Geometry check sheet. Reference: the model listing, model coordinates, mm. Coordinates: 2 decimals unless noted, no trailing zeros. Order: outer loops, then holes, each group sorted by start corner. A loop starts at its lowest first (then second) coordinate and runs counter-clockwise, first axis right, second up.
```python
from build123d import *

# Parameters (mm, degrees)
F2_DEPTH = 12
F3_W     = 392
F3_H     = 368
F3_W_2   = 35
F3_H_2   = 13
F4_DEPTH = 12
F5_R     = 30
F6_R     = 14.99999


# Not quite as in the source:
# - a fillet or chamfer is up to 0.001 mm smaller than in the source, because OpenCascade refuses the exact size
# - a feature names something its author has since deleted; it is built from what else it names


with BuildPart() as f2:
    # F1 (on Front) → F2 (new body)
    with BuildSketch(Plane.XZ):
        Polygon((256, -284), (256, 284), (-256, 284), (-256, -284), (-136, -284), (-136, -254), (136, -254), (136, -284), align=None)
    extrude(amount=F2_DEPTH)

    # F3 (on face) → F4 (cut, through all)
    with BuildSketch(Plane.XZ.offset(12)):
        with Locations((0, 60)):
            Rectangle(F3_W, F3_H)
        with Locations((0, -195.5)):
            Rectangle(F3_W_2, F3_H_2)
    extrude(amount=-F4_DEPTH, mode=Mode.SUBTRACT)

    # F5
    f5_edges = [f2.edges().sort_by_distance(p)[0] for p in [
        (-196, -6, -124),
        (-196, -6, 244),
        (196, -6, 244),
        (196, -6, -124),
    ]]
    fillet(f5_edges, radius=F5_R)

    # F6 (radius 15 in the source; OpenCascade refuses exactly that, so slightly less here)
    f6_edges = [f2.edges().sort_by_distance(p)[0] for p in [
        (-136, -6, -284),
        (-136, -6, -254),
        (136, -6, -284),
        (136, -6, -254),
    ]]
    fillet(f6_edges, radius=F6_R)


solid = f2.part
```
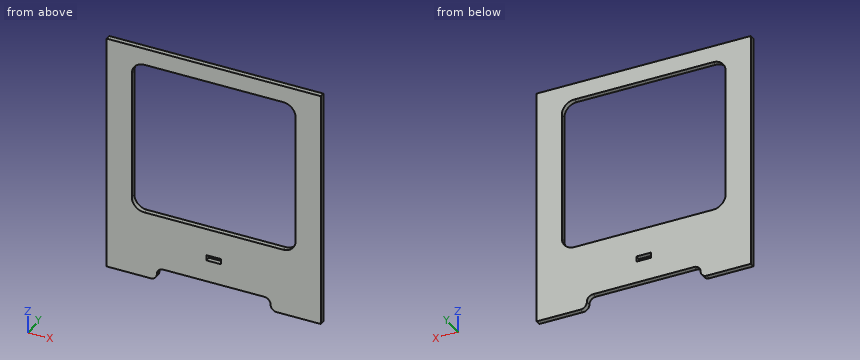
Item 1: Sectioned sample at D-D (x = 1). Record the cut outline in (y, z), and give its area (3 significant figures).
Item 2: Sectioned sample at B-B (y = -7.5). Give the number of separate pieces and of enclosed holes in the cut face, and give its area (3 significant figures).
Item 3: Sectioned sample at A-A (x = 65). Record the cut outline in (y, z), and give its area (3 significant figures).
Item 4: Sectioned sample at C-C (z = 173). Record the cut outline in (x, y).
Item 5: Thickness scan on line 1 along Z through (x, y) = (-18.5, -8); line 2 along X through (y, z) = (-1, 33.5); line 3 along Z through (x, y) = (-10.5, -11). Record the ranges inside material, lowest first.
Geometry check:
1. outline: (-12, -254) - (0, -254) - (0, -202) - (-12, -202) - close; (-12, -189) - (0, -189) - (0, -124) - (-12, -124) - close; (-12, 244) - (0, 244) - (0, 284) - (-12, 284) - close
1. area: 1,880 mm2
2. separate pieces: 1
2. enclosed holes: 2
2. area: 139,000 mm2
3. outline: (-12, -254) - (0, -254) - (0, -124) - (-12, -124) - close; (-12, 244) - (0, 244) - (0, 284) - (-12, 284) - close
3. area: 2,040 mm2
4. outline: (-256, -12) - (-196, -12) - (-196, 0) - (-256, 0) - close; (196, -12) - (256, -12) - (256, 0) - (196, 0) - close
5. line 1: z = -254 to -124, 244 to 284
5. line 2: x = -256 to -196, 196 to 256
5. line 3: z = -254 to -202, -189 to -124, 244 to 284
